from build123d import *

# Parameters (mm, degrees)
F1_DEPTH = 25.4
F2_R     = 6.35
F3_DEPTH = 38.1
F5_DEPTH = 25.4
F7_DEPTH = 25.4


with BuildPart() as f1:
    # F0 (on Front) → F1 (new body)
    with BuildSketch(Plane.XZ):
        Polygon((0, 38.1), (0, 0), (76.2, 0), (76.2, 12.7), (25.4, 12.7), (25.4, 38.1), align=None)
    extrude(amount=F1_DEPTH)

    # F2 (on face) → F3 (cut)
    with BuildSketch(Plane.XY.offset(38.1)):
        with BuildLine():
            ThreePointArc((12.0178175899, -25.4), (4.3513987444, -22.5633729526), (0, -15.6434192037))
            Line((0, -15.6434192037), (0, -25.4))
            Line((0, -25.4), (12.0178175899, -25.4))
        make_face()
        with BuildLine():
            ThreePointArc((0, -9.7565807963), (4.3513987444, -2.8366270474), (12.0178175899, 0))
            Line((12.0178175899, 0), (0, 0))
            Line((0, 0), (0, -9.7565807963))
        make_face()
        with Locations((12.7, -12.7)):
            Circle(F2_R)
    extrude(amount=-F3_DEPTH, mode=Mode.SUBTRACT)

    # F4 (on face) → F5 (cut)
    with BuildSketch(Plane.XY.offset(38.1)):
        with BuildLine():
            ThreePointArc((12.7, 0), (21.6802561211, -3.7197438789), (25.4, -12.7))
            Line((25.4, -12.7), (25.4, 0))
            Line((25.4, 0), (12.7, 0))
        make_face()
        with BuildLine():
            ThreePointArc((25.4, -12.7), (21.6802561211, -21.6802561211), (12.7, -25.4))
            Line((12.7, -25.4), (25.4, -25.4))
            Line((25.4, -25.4), (25.4, -12.7))
        make_face()
    extrude(amount=-F5_DEPTH, mode=Mode.SUBTRACT)

    # F6 (on face) → F7 (cut)
    with BuildSketch(Plane.XY.offset(12.7)):
        with BuildLine():
            Line((63.5, -6.35), (38.1, -6.35))
            ThreePointArc((38.1, -6.35), (31.75, -12.7), (38.1, -19.05))
            Line((38.1, -19.05), (63.5, -19.05))
            Line((63.5, -19.05), (63.5, -6.35))
        make_face()
        with BuildLine():
            ThreePointArc((63.5, -19.05), (69.85, -12.7), (63.5, -6.35))
            Line((63.5, -6.35), (63.5, -19.05))
        make_face()
        with BuildLine():
            ThreePointArc((63.5, 0), (72.4802561211, -3.7197438789), (76.2, -12.7))
            Line((76.2, -12.7), (76.2, 0))
            Line((76.2, 0), (63.5, 0))
        make_face()
        with BuildLine():
            ThreePointArc((76.2, -12.7), (72.4802561211, -21.6802561211), (63.5, -25.4))
            Line((63.5, -25.4), (76.2, -25.4))
            Line((76.2, -25.4), (76.2, -12.7))
        make_face()
    extrude(amount=-F7_DEPTH, mode=Mode.SUBTRACT)


solid = f1.part
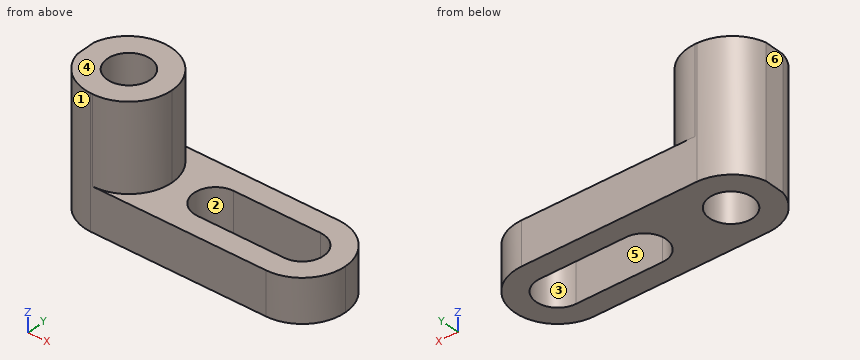
Input: part model. Units: mm. Frame: model coordinates. Face numbers are marked on the shaded views. A direction names the side the tool comes from. Round coordinates to 2 decimals unless told otherwise and drop trailing zeros. Loops run counter-clockwise (first coordinate to the right, second up) from the corner with the lowest first, then second, coordinate; pieces in that order, holes last. Notation, with made-up numbers: (-30, 9) -> (-24, 9) arc R20 ccw to (-24, 38) -> close; hole circle Ø7 at (9, 70). An arc over 180 degrees is marked (long way). Answer as a JSON object with one key per item and string values. Group by question number.
1) Section query A-A on x = 46. Output: boundary loops of the cut face in (y, z).
2) Section query B-B on z = 11. Output: boundary loops of the cut face in (x, y).
3) Reachability of the marked faces 1 and 2 from +Z, -Z, +X, -X, +Y, -Y: full face, straight path, thin tool, end or side. Return the list, or none.
4) Draft query along X for the marked faces 3, 4, 5 and 6. Return one class per face: +X half, -X half, draft (parallel to the pull), parting line (faces both ways), or undercut.
5) Section query C-C on y = -16.5. Output: boundary loops of the cut face in (x, z).
6) Pin query (flat end, axial travel): pin 1 (6 mm diameter, centred on y = -15, z = 13, fed in from +X); pin 2 (3 mm diameter, centred on x = 64, z = 14.5, fed in from -Y); pin 3 (4 mm diameter, centred on y = -18.5, z = 26, fed in from +X); pin 4 (10 mm diameter, centred on y = -3, z = 26, fed in from -X). Return the tip coordinate at first contact, or that it passes through.
7) Ray query, L1, parallel to Y at x = 12.7, z = 11; L2, parallel to Z at x = 34.5, y = -2.75; L3, parallel to X at y = -12, z = 4. Return the intervals inside material, ascending.
8) Section query D-D on z = 23. Output: boundary loops of the cut face in (x, y), plus the area to 3 significant figures.
Reply:
{
 "1": {"outline": "(-25.4, 0) -> (-19.05, 0) -> (-19.05, 12.7) -> (-25.4, 12.7) -> close; (-6.35, 0) -> (0, 0) -> (0, 12.7) -> (-6.35, 12.7) -> close"},
 "2": {"outline": "(0, -15.64) arc R12.7 ccw to (12.02, -25.4) -> (63.5, -25.4) arc R12.7 ccw to (63.5, 0) -> (12.02, 0) arc R12.7 ccw to (0, -9.76) -> close; hole circle Ø12.7 at (12.7, -12.7); hole (38.1, -19.05) -> (63.5, -19.05) arc R6.35 ccw to (63.5, -6.35) -> (38.1, -6.35) arc R6.35 ccw to start"},
 "3": {"face 1": "+Z, -Z, -X, -Y", "face 2": "+Z, -Z"},
 "4": {"face 3": "undercut", "face 4": "draft", "face 5": "undercut", "face 6": "-X half"},
 "5": {"outline": "(0.24, 0) -> (7.61, 0) -> (7.61, 38.1) -> (0.24, 38.1) -> close; (17.79, 0) -> (33.01, 0) -> (33.01, 12.7) -> (24.82, 12.7) -> (24.82, 38.1) -> (17.79, 38.1) -> close; (68.59, 0) -> (75.62, 0) -> (75.62, 12.7) -> (68.59, 12.7) -> close"},
 "6": {"pin 1": "stops at x = 76.2", "pin 2": "passes through", "pin 3": "stops at x = 24.82", "pin 4": "stops at x = 0.56"},
 "7": {"L1": "y = -25.4 to -19.05, -6.35 to 0", "L2": "z = 0 to 12.7", "L3": "x = 0 to 6.39, 19.01 to 31.79, 69.81 to 76.18"},
 "8": {"outline": "(0, -15.64) arc R12.7 ccw to (12.02, -25.4) -> (12.7, -25.4) arc R12.7 ccw to (12.7, 0) -> (12.02, 0) arc R12.7 ccw to (0, -9.76) -> close; hole circle Ø12.7 at (12.7, -12.7)", "area": "388 mm2"}
}
